For this review, take the finished solid that the model builds, in its own axes (mm). A direction names the side the tool comes from. Round coordinates to 2 decimals unless told otherwise and drop trailing zeros. Loops run counter-clockwise (first coordinate to the right, second up) from the corner with the lowest first, then second, coordinate; pieces in that order, holes last.
1) Mouldability with a two-part tool opening along X and no side actions: class faces 1 (the flat face through (41.536, -0.036, -49.453)), 2 (the flat face through (-0.036, -52.595, -71.436)), 3 (the flat face through (24, 0, -78.258)) as pulls with the +X half, pulls with the -X half, needs draft (parallel to the pull), parting line crosses it, or undercut.
2) Wall thickness on L1, parallel to Y at x = 0, z = -13; L2, parallel to X at y = 0, z = -79; L3, parallel to X at y = 0, z = -78.75: over which ranges is each line inside the solid? List them lowest first.
3) Take a section at B-B (z = -60.5). State the section outline as (x, y) points, then the cut area to 3 significant figures.
4) Insertion check: pin 1 (5 mm diameter, centred on x = 25, y = 1, fed in from -Z); pin 2 (24.5 mm diameter, centred on y = -45, z = -59, fed in from +X); pin 3 (3 mm diameter, centred on y = 22.5, z = -13.5, fed in from -X). Each pin has a flat end and moves straight along its axis. Give the tip position at first contact, or say it passes through.
5) Tool access review of faces 4 (the cylindrical face through (-0.794, 6.044, -12.522)), 5 (the flat face through (0, 47, -79.101)), 6 (the cylindrical face through (-0.668, 18.854, -78.774)): name each direction out of +Z, -Z, +X, -X, +Y, -Y from which nothing blocks a thin tool from reaching the whole face with its end or side.
6) Take a section at A-A (z = -7.5). State the section outline as (x, y) points.
```python
from build123d import *

# Parameters (mm, degrees)
F0_W     = 3.4201149829
F0_H     = 19.8584441096
F0_W_2   = 2.4988718903
F0_W_3   = 1.865520142
F0_W_4   = 2.0727999508
F0_W_5   = 2.0727985539
F0_W_6   = 2.0727962255
F0_W_7   = 2.4873549119
F0_W_8   = 2.9019191861
F0_W_9   = 2.4873595685
F0_W_10  = 2.2800769657
F0_W_11  = 2.9019173235
F0_W_12  = 2.5449345174
F0_W_13  = 1.6582384706
F0_W_14  = 2.0152203453
F3_DEPTH = 2.54
F4_COUNT = 4
F5_R     = 5.1308
F6_DEPTH = 1.016
F7_R     = 6.096
F8_DEPTH = 25.4


with BuildPart() as f1:
    # F0 (on Front) → F1 (revolve)
    with BuildSketch(Plane.XZ):
        Polygon((-35.56, -79.2744270182), (0, -79.2744270182), (0, -19.8584441096), (-3.4201149829, -19.8584441096), (-5.2856351249, -19.8584441096), (-7.3584336787, -19.8584441096), (-9.8457885906, -19.8584441096), (-12.3331481591, -19.8584441096), (-15.2350654826, -19.8584441096), (-17.78, -19.8584441096), (-19.7952203453, -19.8584441096), (-21.4534588158, -19.8584441096), (-23.7335357815, -19.8584441096), (-26.0136127472, -19.8584441096), (-28.9155319333, -19.8584441096), (-30.9883281589, -19.8584441096), (-33.0611281097, -19.8584441096), (-35.56, -19.8584441096), align=None)
        with Locations((-1.7100574914, -9.9292220548)):
            Rectangle(F0_W, F0_H)
        with Locations((-34.3105640548, -9.9292220548)):
            Rectangle(F0_W_2, F0_H)
        with Locations((-4.3528750539, -9.9292220548)):
            Rectangle(F0_W_3, F0_H)
        with Locations((-32.0247281343, -9.9292220548)):
            Rectangle(F0_W_4, F0_H)
        with Locations((-6.3220344018, -9.9292220548)):
            Rectangle(F0_W_5, F0_H)
        with Locations((-29.9519300461, -9.9292220548)):
            Rectangle(F0_W_6, F0_H)
        with Locations((-8.6021111347, -9.9292220548)):
            Rectangle(F0_W_7, F0_H)
        with Locations((-27.4645723403, -9.9292220548)):
            Rectangle(F0_W_8, F0_H)
        with Locations((-11.0894683748, -9.9292220548)):
            Rectangle(F0_W_9, F0_H)
        with Locations((-24.8735742643, -9.9292220548)):
            Rectangle(F0_W_10, F0_H)
        with Locations((-13.7841068208, -9.9292220548)):
            Rectangle(F0_W_11, F0_H)
        with Locations((-22.5934972987, -9.9292220548)):
            Rectangle(F0_W_10, F0_H)
        with Locations((-16.5075327413, -9.9292220548)):
            Rectangle(F0_W_12, F0_H)
        with Locations((-20.6243395805, -9.9292220548)):
            Rectangle(F0_W_13, F0_H)
        with Locations((-18.7876101726, -9.9292220548)):
            Rectangle(F0_W_14, F0_H)
    revolve(axis=Axis((0, 0, -38.7951713055), (0, 0, -1)))

    # F2 (on Front) → F3 (join, symmetric)
    with BuildSketch(Plane.XZ):
        Polygon((35.4841057915, -36.6654805839), (35.1339280605, -79.1006311774), (47.1561551094, -79.1006311774), (47.1561551094, -63.5546445847), (35.755764693, -34.9500365555), (35.4887494468, -34.563057843), align=None)
        Polygon((47.1561551094, -63.5546445847), (47.1561551094, -79.1006311774), (57.8828832321, -79.1006311774), align=None)
    extrude(amount=F3_DEPTH, both=True)

    # F4: F1 ×4 about axis
    f4_axis = Axis((0, 0, -38.7951713055), (0, 0, -1))


with BuildPart() as f1_1:
    add(f1.part)
    for i in range(1, F4_COUNT):
        add(f1.part.rotate(f4_axis, i * 360 / F4_COUNT))

    # F5 (on face) → F6 (cut)
    with BuildSketch(Plane(origin=(0, 0, -79.2744270182), x_dir=(1, 0, 0), z_dir=(0, 0, -1))):
        Circle(F5_R)
        with Locations((-23.9408165216, 0)):
            Circle(F5_R)
        with Locations((0, 23.9408165216)):
            Circle(F5_R)
        with Locations((23.9408165216, 0)):
            Circle(F5_R)
        with Locations((0, -23.9408165216)):
            Circle(F5_R)
    extrude(amount=-F6_DEPTH, mode=Mode.SUBTRACT)

    # F7 (on Top) → F8 (cut)
    with BuildSketch(Plane.XY):
        Circle(F7_R)
    extrude(amount=-F8_DEPTH, mode=Mode.SUBTRACT)


solid = f1_1.part
```
Response:
1. face 1: pulls with the +X half
1. face 2: needs draft
1. face 3: undercut
2. L1: y = -35.56 to -6.1, 6.1 to 35.56
2. L2: x = -57.81 to -29.07, -18.81 to -5.13, 5.13 to 18.81, 29.07 to 57.81
2. L3: x = -57.64 to -29.07, -18.81 to -5.13, 5.13 to 18.81, 29.07 to 57.64
3. outline: (-45.94, -2.54) - (-35.47, -2.54) arc R35.56 ccw to (-2.54, -35.47) - (-2.54, -45.94) - (2.54, -45.94) - (2.54, -35.47) arc R35.56 ccw to (35.47, -2.54) - (45.94, -2.54) - (45.94, 2.54) - (35.47, 2.54) arc R35.56 ccw to (2.54, 35.47) - (2.54, 45.94) - (-2.54, 45.94) - (-2.54, 35.47) arc R35.56 ccw to (-35.47, 2.54) - (-45.94, 2.54) - close
3. area: 4,180 mm2
4. pin 1: stops at z = -78.26
4. pin 2: stops at x = 13.85
4. pin 3: stops at x = -28.7
5. face 4: +Z
5. face 5: -Z, +X, -X, +Y
5. face 6: -Z
6. outline: circle Ø71.12 at (0, 0); hole circle Ø12.19 at (0, 0)
